from build123d import *

# Parameters (mm, degrees)
SKETCH1_R           = 6
SKETCH1_R_2         = 3
BOSS_EXTRUDE1_DEPTH = 11
SKETCH2_R           = 1.5
CUT_EXTRUDE1_DEPTH  = 14.892443989
SKETCH3_R           = 6
BOSS_EXTRUDE2_DEPTH = 4
BOSS_EXTRUDE3_DEPTH = 7
SKETCH5_R           = 3
BOSS_EXTRUDE6_DEPTH = 14
SKETCH7_R           = 2.5
BOSS_EXTRUDE7_DEPTH = 5
FILLET1_R           = 0.5


with BuildPart() as part:
    # Sketch1 → Boss-Extrude1 (new body)
    with BuildSketch(Plane.XY):
        Circle(SKETCH1_R)
        Circle(SKETCH1_R_2, mode=Mode.SUBTRACT)
    extrude(amount=BOSS_EXTRUDE1_DEPTH)

    # Sketch2 → Cut-Extrude1 (cut, through all)
    with BuildSketch(Plane(origin=(0, 0, 0), x_dir=(1, 0, 0), z_dir=(0, 1, 0))):
        with Locations(Location((0, -6, 0), (0, 0, 90))):
            Circle(SKETCH2_R)
    extrude(amount=CUT_EXTRUDE1_DEPTH, mode=Mode.SUBTRACT)

    # Sketch3 → Boss-Extrude2 (add)
    with BuildSketch(Plane.XY.offset(11)):
        Circle(SKETCH3_R)
    extrude(amount=BOSS_EXTRUDE2_DEPTH)

    # Sketch4 → Boss-Extrude3 (add)
    with BuildSketch(Plane.XY.offset(15)):
        with BuildLine():
            Line((-1.658312395, 2.5), (1.658312395, 2.5))
            ThreePointArc((1.658312395, 2.5), (0, -3), (-1.658312395, 2.5))
        make_face()
    extrude(amount=BOSS_EXTRUDE3_DEPTH)

    # Sketch5 → Boss-Extrude6 (add)
    with BuildSketch(Plane.XY.offset(22)):
        Circle(SKETCH5_R)
    extrude(amount=BOSS_EXTRUDE6_DEPTH)

    # Sketch7 → Boss-Extrude7 (add)
    with BuildSketch(Plane.XY.offset(36)):
        Circle(SKETCH7_R)
    extrude(amount=BOSS_EXTRUDE7_DEPTH)

    # Fillet1
    fillet1_edges = [part.edges().sort_by_distance(p)[0] for p in [
        (0, -3, 15),
    ]]
    fillet(fillet1_edges, radius=FILLET1_R)


solid = part.part
The model under review builds one solid part; all positions refer to its coordinate system, in mm. A direction names the side the tool comes from. Give positions to 0.01 mm unless a question says otherwise; leave off trailing zeros. Write each loop counter-clockwise with the first axis right and the second up, starting at its lowest first coordinate (ties: lowest second). Pieces come first, ordered by that corner, then holes. Notation, with made-up numbers: M -15.5,53 L 30.5,53 A21 ccw 30.5,82 Z; hole C -15.5,25 d2. An arc over 180 degrees is marked long. One line per question, with ' | ' between items. Start each with the question number.
Item 1: Wall thickness on line 1 (Y direction, x = 0, z = 4.25); line 2 (X direction, y = 2.5, z = 34); line 3 (Z direction, x = -1.25, y = -3.5): over which ranges is each line inside the solid? List them lowest first. Write a range as from..to.
Item 2: We need section C-C on z = 34.5. Write out the cut boundary in (x, y), plus the area to 3 significant figures.
Item 3: For faces 1 (the flat face through (-2, 2, 36)), 2 (the flat face through (0, 2.5, 18)), 3 (the cylindrical face through (-0.65, -2.93, 5.42)), list the 3-axis set-ups (+Z, -Z, +X, -X, +Y, -Y) from which the entire face can be reached by the end or side of a thin tool; tool diameter is ignored.
Item 4: We need section A-A on x = 0. Write out the cut boundary in (y, z), plus the area to 3 significant figures.
Item 5: For pin 1 (5 mm diameter, centred on x = -0.5, y = -1, fed in from -Z); pin 2 (1 mm diameter, centred on y = -1, z = 29.5, fed in from -X); pin 3 (5.5 mm diameter, centred on x = 0, y = 0, fed in from -Z); pin 4 (2.5 mm diameter, centred on x = 0, z = 6, fed in from +Y), all flat-tipped, find the tip position at first contact; note any pin that passes through.
Item 6: We need section D-D on x = -4. Write out the cut boundary in (y, z), plus the area to 3 significant figures.
Item 7: We need section B-B on z = 18. Write out the cut boundary in (x, y), plus the area to 3 significant figures.
Item 8: Draft analysis for pull direction Z (two halves, no side actions). For faces 4 (the flat face through (0, 0, 41)), 5 (the cylindrical face through (0.575, 4.278, 4.614)), 6 (the cylindrical face through (-0.54, -2.44, 38.47)), state which applies: released by +Z, released by -Z, zero draft, split by the parting line, or undercut.
Results found:
1) line 1: y = -6..-3, 3..6 | line 2: x = -1.66..1.66 | line 3: z = 0..15
2) outline: C 0,0 d6 | area: 28.3 mm2
3) face 1: +Z | face 2: +X, -X, +Y | face 3: -Z
4) outline: M -6,0 L -3,0 L -3,11 L 3,11 L 3,7.5 L 6,7.5 L 6,15 L 2.5,15 L 2.5,22 L 3,22 L 3,36 L 2.5,36 L 2.5,41 L -2.5,41 L -2.5,36 L -3,36 L -3,15.5 A0.5 cw -3.5,15 L -6,15 Z; M 3,0 L 6,0 L 6,4.5 L 3,4.5 Z | area: 253 mm2
5) pin 1: stops at z = 0 | pin 2: stops at x = -2.96 | pin 3: stops at z = 11 | pin 4: stops at y = -2.73
6) outline: M -4.47,0 L 4.47,0 L 4.47,15 L -4.47,15 Z | area: 134 mm2
7) outline: M -1.66,2.5 A3 ccw long 1.66,2.5 Z | area: 27.1 mm2
8) face 4: released by +Z | face 5: undercut | face 6: zero draft
